from build123d import *

# Parameters (mm, degrees)
SKETCH1_W           = 20
SKETCH1_H           = 20
BOSS_EXTRUDE1_DEPTH = 5
SKETCH4_W           = 0.5
SKETCH4_H           = 0.5
CUT_EXTRUDE1_DEPTH  = 7
FILLET1_R           = 2
SKETCH5_W           = 5
SKETCH5_H           = 5
CUT_EXTRUDE2_DEPTH  = 2.5
SKETCH6_R           = 1
CUT_EXTRUDE3_DEPTH  = 3
FILLET2_R           = 0.5


with BuildPart() as part:
    # Sketch1 → Boss-Extrude1 (new body)
    with BuildSketch(Plane(origin=(0, 0, 0), x_dir=(1, 0, 0), z_dir=(0, 1, 0))):
        with Locations((10, 10)):
            Rectangle(SKETCH1_W, SKETCH1_H)
    extrude(amount=BOSS_EXTRUDE1_DEPTH)

    # Sketch3 → Cut-Revolve3 (revolve, cut)
    with BuildSketch(Plane(origin=(10, 0, 0), x_dir=(0, 0, -1), z_dir=(1, 0, 0))):
        Polygon((10, 0.3), (10, 5), (5, 5), align=None)
    revolve(axis=Axis((10, 5, -10), (0, -1, 0)), mode=Mode.SUBTRACT)

    # Sketch4 → Cut-Extrude1 (cut)
    with BuildSketch(Plane(origin=(0, 5, 0), x_dir=(1, 0, 0), z_dir=(0, 1, 0))):
        with Locations((10, 10)):
            Rectangle(SKETCH4_W, SKETCH4_H)
    extrude(amount=-CUT_EXTRUDE1_DEPTH, mode=Mode.SUBTRACT)

    # Fillet1
    fillet1_edges = [part.edges().sort_by_distance(p)[0] for p in [
        (10, 5, -15),
    ]]
    fillet(fillet1_edges, radius=FILLET1_R)

    # Sketch5 → Cut-Extrude2 (cut)
    with BuildSketch(Plane(origin=(0, 0, 0), x_dir=(-1, 0, 0), z_dir=(0, -1, 0))):
        with Locations((-17.5, 17.5)):
            Rectangle(SKETCH5_W, SKETCH5_H)
        with Locations((-2.5, 17.5)):
            Rectangle(SKETCH5_W, SKETCH5_H)
        with Locations((-17.5, 2.5)):
            Rectangle(SKETCH5_W, SKETCH5_H)
        with Locations((-2.5, 2.5)):
            Rectangle(SKETCH5_W, SKETCH5_H)
    extrude(amount=-CUT_EXTRUDE2_DEPTH, mode=Mode.SUBTRACT)

    # Sketch6 → Cut-Extrude3 (cut)
    with BuildSketch(Plane(origin=(0, 5, 0), x_dir=(1, 0, 0), z_dir=(0, 1, 0))):
        with Locations((17.966640292, 2.023795915)):
            Circle(SKETCH6_R)
        with Locations((17.5, 17.5)):
            Circle(SKETCH6_R)
        with Locations((2.5, 17.5)):
            Circle(SKETCH6_R)
        with Locations((2.5, 2.5)):
            Circle(SKETCH6_R)
    extrude(amount=-CUT_EXTRUDE3_DEPTH, mode=Mode.SUBTRACT)

    # Fillet2
    fillet2_edges = [part.edges().sort_by_distance(p)[0] for p in [
        (16.5, 5, -17.5),
        (1.5, 5, -17.5),
        (1.5, 5, -2.5),
        (16.966640292, 5, -2.023795915),
    ]]
    fillet(fillet2_edges, radius=FILLET2_R)


solid = part.part
Input: part model. Units: mm. Frame: model coordinates. A direction names the side the tool comes from. Coordinates: 2 decimals unless noted, no trailing zeros. Loops run counter-clockwise (first coordinate to the right, second up) from the corner with the lowest first, then second, coordinate; pieces in that order, holes last.
(1) Material intervals for probe 1 along Z at (x, y) = (2.5, 3); probe 2 along X at (y, z) = (3.05, -17.5); probe 3 along X at (y, z) = (3.5, -2.5), sorted ascending.
(2) First-contact query: pin 1 Ø2.5 at (x, z) = (2.5, -2.5) entering from -Y; pin 2 Ø0.8 at (x, y) = (17.5, 0.5) entering from -Z; pin 3 Ø3 at (y, z) = (0.5, -18) entering from +X. Flat tips, straight axial feed; report the tip coordinate or a pass-through.
(3) Set-up query: faces 1 (the face through (1, 2.5, -3)), 2 (the face through (15, 1, -2)), 3 (the face through (16, 2.5, -18)), 4 (the face through (5, 1, -17)). Return all of +Z, -Z, +X, -X, +Y, -Y with unobstructed straight access to the full face (end or side cutting, diameter ignored); none if empty.
(4) Section C-C on z = -17.5. Return the cut outline in (x, y), then the cut area to 3 significant figures.
(5) Section B-B on x = 2.5. Return the cut outline in (y, z), then the cut area to 3 significant figures.
(6) Section D-D on x = 10. Return the cut outline in (y, z) (3 decimals).
(7) Pull-direction query (X, two-part tool) for faces 5 (the face through (18, 1, -5)), 6 (the face through (15, 1, -17)), 7 (the face through (17.96, 3.51, -16.61)); classes: released by +X, released by -X, zero draft, split by the parting line, or undercut.
(8) Section A-A on z = -10. Return the cut outline in (x, y) (3 decimals), then the cut area to 3 significant figures.
Data:
1. probe 1: z = -20 to -18.5, -16.5 to -3.5, -1.5 to 0
1. probe 2: x = 0 to 1.5, 3.5 to 16.5, 18.5 to 20
1. probe 3: x = 0 to 1.5, 3.5 to 17.09, 18.85 to 20
2. pin 1: stops at y = 2.5
2. pin 2: stops at z = -15
2. pin 3: stops at x = 15
3. face 1: +Z, -X, -Y
3. face 2: +Z, +X, -Y
3. face 3: -Z, +X, -Y
3. face 4: -Z, -X, -Y
4. outline: (0, 2.5) - (1.5, 2.5) - (1.5, 4.5) arc R0.5 ccw to (1, 5) - (0, 5) - close; (3.5, 2.5) - (5, 2.5) - (5, 0) - (15, 0) - (15, 2.5) - (16.5, 2.5) - (16.5, 4.5) arc R0.5 ccw to (16, 5) - (4, 5) arc R0.5 ccw to (3.5, 4.5) - close; (18.5, 2.5) - (20, 2.5) - (20, 5) - (19, 5) arc R0.5 ccw to (18.5, 4.5) - close
4. area: 64.8 mm2
5. outline: (0, -15) - (2.5, -15) - (2.5, -16.5) - (4.5, -16.5) arc R0.5 ccw to (5, -16) - (5, -4) arc R0.5 ccw to (4.5, -3.5) - (2.5, -3.5) - (2.5, -5) - (0, -5) - close; (2.5, -20) - (5, -20) - (5, -19) arc R0.5 ccw to (4.5, -18.5) - (2.5, -18.5) - close; (2.5, -1.5) - (4.5, -1.5) arc R0.5 ccw to (5, -1) - (5, 0) - (2.5, 0) - close
5. area: 64.8 mm2
6. outline: (0, -20) - (5, -20) - (5, -15.792) arc R2 ccw to (4.457, -14.423) - (0.535, -10.25) - (0, -10.25) - close; (0, -9.75) - (0.535, -9.75) - (4.457, -5.577) arc R2 ccw to (5, -4.208) - (5, 0) - (0, 0) - close
7. face 5: zero draft
7. face 6: released by +X
7. face 7: undercut
8. outline: (0, 0) - (9.75, 0) - (9.75, 0.535) - (5.577, 4.457) arc R2 ccw to (4.208, 5) - (0, 5) - close; (10.25, 0) - (20, 0) - (20, 5) - (15.792, 5) arc R2 ccw to (14.423, 4.457) - (10.25, 0.535) - close
8. area: 76.1 mm2
